Can you work these out from the model? Positions are in its coordinate system, mm. Face numbers are marked on the shaded views. Give positions to 0.01 mm unless a question says otherwise; leave off trailing zeros. Order: outer loops, then holes, each group sorted by start corner. A loop starts at its lowest first (then second) coordinate and runs counter-clockwise, first axis right, second up. Notation, with made-up numbers: M -12.75,-31.75 L 34.25,-31.75 A30 ccw 34.25,-1.75 Z; hole C 35,10 d6. An arc over 180 degrees is marked long. Write each question's results on one line, items separated by ' | '.
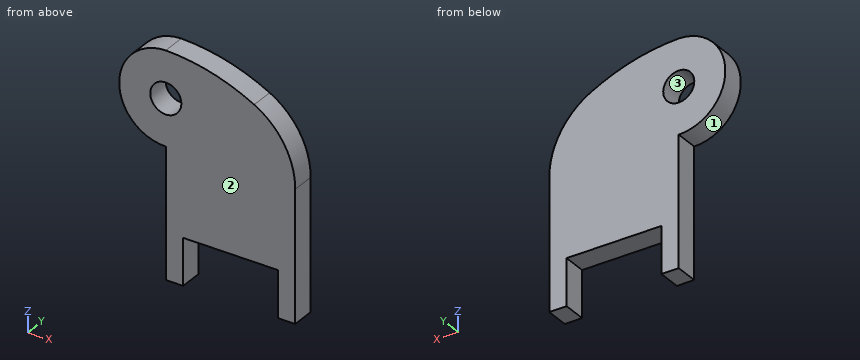
from build123d import *

# Parameters (mm, degrees)
SKETCH_1_R      = 2
EXTRUDE_1_DEPTH = 3
FILLET_1_R      = 10


with BuildPart() as part:
    # 草图1 → 凸台-拉伸1 (new body)
    with BuildSketch(Plane(origin=(0, 0, 0), x_dir=(1, 0, 0), z_dir=(0, 1, 0))):
        with BuildLine():
            Line((2.233333333, 0), (0, 0))
            Line((0, 0), (0, -16.666666667))
            ThreePointArc((0, -16.666666667), (-6, -22.666666667), (0, -28.666666667))
            add(Edge.make_bspline(
                [(0, -28.666666667), (9.212627714, -28.392938173), (16.666666667, -22)],
                knots=[0, 0, 0, 1, 1, 1], degree=2))
            Line((16.666666667, -22), (16.666666667, 0))
            Line((16.666666667, 0), (14.433333333, 0))
            Line((14.433333333, 0), (14.433333333, -6))
            Line((14.433333333, -6), (2.233333333, -6))
            Line((2.233333333, -6), (2.233333333, 0))
        make_face()
        with Locations(Location((0, -22.666666667, 0), (0, 0, 270))):
            Circle(SKETCH_1_R, mode=Mode.SUBTRACT)
    extrude(amount=EXTRUDE_1_DEPTH)

    # 圆角1
    fillet_1_edges = [part.edges().sort_by_distance(p)[0] for p in [
        (16.666666667, 1.5, 22),
    ]]
    fillet(fillet_1_edges, radius=FILLET_1_R)


solid = part.part
(1) Imagine slicing it at B-B, the plane x = -4.5. Write out the boundary of the cut face in (y, z).
Data:
outline: M 0,18.7 L 3,18.7 L 3,26.64 L 0,26.64 Z
(2) Will these pins go through, and if not, where does the flat tip stop? P1, Ø1.5, axis at x = 13, y = 2.5, coming from the +Z side; P2, Ø1, axis at x = 1, y = 2.5, coming from the +Z side.
Data:
P1: stops at z = 25.12 | P2: stops at z = 28.65
(3) We'd pull the mould along X, two halves only. Please class the marked faces 1, 2 and 3: +X half, -X half, draft (parallel to the pull), parting line (faces both ways), or undercut.
Data:
face 1: -X half | face 2: draft | face 3: undercut
(4) I need wall thicknesses on L1, parallel to X at y = 0.25, z = 2.25; L2, parallel to X at y = 0.9, z = 6.25; L3, parallel to X at y = 0.6, z = 22.75. Which ranges of each line are inside material? Lowest first, please. Write a range as from..to.
Data:
L1: x = 0..2.23, 14.43..16.67 | L2: x = 0..16.67 | L3: x = -6..-2, 2..14.72
(5) Imagine slicing it at A-A, the plane z = 5. Write out the boundary of the cut face in (x, y), plus the area to 3 significant figures.
Data:
outline: M 0,0 L 2.23,0 L 2.23,3 L 0,3 Z; M 14.43,0 L 16.67,0 L 16.67,3 L 14.43,3 Z | area: 13.4 mm2
